Read the model definition and answer for the solid it produces. Units are mm, in the model's axes. A direction names the side the tool comes from. Coordinates: 2 decimals unless noted, no trailing zeros. Order: outer loops, then holes, each group sorted by start corner. A loop starts at its lowest first (then second) coordinate and runs counter-clockwise, first axis right, second up.
Autodesk Fusion 360 part; units mm, degrees
sketch "Sketch1" plane through (0, 0, 0) normal (0, 0, 1) x (1, 0, 0)
  line L0 (9, 7.5) -> (-9, 7.5)
  line L1 (-9, 7.5) -> (-9, -7.5)
  line L2 (-9, -7.5) -> (9, -7.5)
  line L3 (9, -7.5) -> (9, 7.5)
  line L4 (9, 7.5) -> (-9, -7.5) construction
  line L5 (-9, 7.5) -> (9, -7.5) construction
  circle A0 centre (-3.5, 0) radius 1.75
  circle A1 centre (-3.5, 0) radius 3
  line L6 (9, -2.8) -> (-9, -2.8)
  line L7 (-9, -2.8) -> (-9, 2.8)
  line L8 (-9, 2.8) -> (9, 2.8)
  line L9 (9, 2.8) -> (9, -2.8)
  line L10 (9, -2.8) -> (-9, 2.8) construction
  line L11 (-9, -2.8) -> (9, 2.8) construction
  dimension "d1" = 18
  dimension "d2" = 15
  dimension "d5" = 3.5
  dimension "d6" = 6
  dimension "d9" = 5.6
  dimension "d12" = 3.5
extrude "Extrude1" add sketch "Sketch1" along normal blind 2
extrude "Extrude2" add sketch "Sketch1" along normal blind 4 contours L0 L1 L3 A1 L8 | L3 A1 L6 L8 L9 | L1 A1 L6 L7 L8 | L1 L2 L3 A1 L6
extrude "Extrude3" add sketch "Sketch1" against normal blind 1 contours L3 A1 L6 L8 L9 | L1 A1 L6 L7 L8 | A1 L6 L8
sketch "Sketch2" plane through (9, 0, 0) normal (1, 0, 0) x (0, 1, 0)
  line L0 (-7.5, 0) -> (-2.8, 0)
  line L1 (-2.8, 0) -> (-2.8, -1)
  line L2 (-2.8, -1) -> (2.8, -1)
  line L3 (2.8, -1) -> (2.8, 0)
  line L4 (2.8, 0) -> (7.5, 0)
  line L5 (7.5, 0) -> (7.5, 4)
  line L6 (7.5, 4) -> (-7.5, 4)
  line L7 (-7.5, 4) -> (-7.5, 0)
  circle A0 centre (0, 5) radius 2.25
  circle A1 centre (0, 5) radius 4.45
  line L8 (-7.5, 0) -> (7.5, 0)
  dimension "d13" = 4.5
  dimension "d14" = 2.2
  dimension "d18" = 5
extrude "Extrude4" cut sketch "Sketch2" against normal blind 3.5 from surface at -3.5 contours L6 A0 A1 picked at (-0.2762, 1.3019)
chamfer "Chamfer1" distance 1.2 angle 45 1 edges at (-5.1316, 0.6328, 2)
fillet "Fillet1" radius 2 4 edges at (-9, -7.5, 2) (9, -7.5, 2) (9, 7.5, 2) (-9, 7.5, 2)
chamfer "Chamfer2" distance 1 angle 45 2 edges at (-9, 0, -1) (9, 0, -1)
Q1. Straight lines are drawn through the part: L1, parallel to X at y = 0, z = 2.5; L2, parallel to Y at x = -3.5, z = 0.25; L3, parallel to X at y = 3.5, z = 2.55. For each, find the intervals that lie inside material, in ascending order.
Q2. The part is cut by section B-B, the plane x = -3.5. Determine the outline of the cut face in (y, z), then the cut area to 3 significant figures.
Q3. The part is cut by section D-D, the plane z = 2.3. Determine the outline of the cut face in (x, y).
Q4. The part is cut by section C-C, the plane z = -0.25. Determine the outline of the cut face in (x, y), then the cut area to 3 significant figures.
Q5. The part is cut by section A-A, the plane y = 0. Determine the outline of the cut face in (x, z).
Q6. Each of these flat-tipped pins is pushed along its axis until it touches: P1, Ø4, axis at x = -3.5, y = 0, coming from the +Z side; P2, Ø4, axis at x = 2.5, y = 5, coming from the -Z side. Where does it stop, or does it pass through?
Q7. Determine the mould class of faces 1 (the cylindrical face through (3.77, -0.03, 2.75)), 2 (the cylindrical face through (-8.4, 6.93, 2.03)), 3 (the flat face through (0, 5, 0)), 4 (the cylindrical face through (3.77, -0.08, 0.55)) for opening direction X: +X half, -X half, draft (parallel to the pull), parting line (faces both ways), or undercut.
Q8. Which of the six approach directions +Z, -Z, +X, -X, +Y, -Y give full straight-line access (tool end or side, diameter ignored) to faces 5 (the flat face through (0, -5, 0)), 6 (the flat face through (-0.1, 2.8, -0.5)), 7 (the cylindrical face through (-5.9, 1.8, 3)), 8 (the flat face through (2, 0, 2)), 9 (the cylindrical face through (8.43, -6.9, 1.97))?
Computed values:
1. L1: x = -9 to -6.5, -0.5 to 2, 5.5 to 9
1. L2: y = -7.5 to -1.75, 1.75 to 7.5
1. L3: x = -9 to 2, 5.5 to 9
2. outline: (-7.5, 0) - (-2.8, 0) - (-2.8, -1) - (-1.75, -1) - (-1.75, 0.8) - (-2.95, 2) - (-3, 2) - (-3, 4) - (-7.5, 4) - close; (1.75, -1) - (2.8, -1) - (2.8, 0) - (7.5, 0) - (7.5, 4) - (3, 4) - (3, 2) - (2.95, 2) - (1.75, 0.8) - close
2. area: 41.7 mm2
3. outline: (-9, -5.5) arc R2 ccw to (-7, -7.5) - (7, -7.5) arc R2 ccw to (9, -5.5) - (9, 5.5) arc R2 ccw to (7, 7.5) - (-7, 7.5) arc R2 ccw to (-9, 5.5) - close; hole circle Ø6 at (-3.5, 0); hole (2, -3.54) - (5.5, -3.54) - (5.5, 3.54) - (2, 3.54) - close
4. outline: (-8.75, -2.8) - (8.75, -2.8) - (8.75, 2.8) - (-8.75, 2.8) - close; hole circle Ø3.5 at (-3.5, 0)
4. area: 88.4 mm2
5. outline: (-9, 0) - (-8, -1) - (-5.25, -1) - (-5.25, 0.8) - (-6.45, 2) - (-6.5, 2) - (-6.5, 4) - (-9, 4) - close; (-1.75, -1) - (8, -1) - (9, 0) - (9, 4) - (-0.5, 4) - (-0.5, 2) - (-0.55, 2) - (-1.75, 0.8) - close; hole (2, 0.55) - (5.5, 0.55) - (5.5, 2.75) - (2, 2.75) - close
6. P1: stops at z = 1.05
6. P2: stops at z = 0
7. face 1: undercut
7. face 2: -X half
7. face 3: draft
7. face 4: undercut
8. face 5: -Z, +X, -X, -Y
8. face 6: -Z, +X, -X, +Y
8. face 7: +Z
8. face 8: none
8. face 9: +Z, -Z, +X, -Y
